```python
from build123d import *

# Parameters (mm, degrees)
SKETCH1_W           = 65.8
SKETCH1_H           = 130
BOSS_EXTRUDE1_DEPTH = 11.4
CUT_EXTRUDE1_DEPTH  = 94.191201301
FILLET1_R           = 11
SKETCH3_R           = 5.5
SKETCH3_R_2         = 2.75
CUT_EXTRUDE2_DEPTH  = 1
SKETCH4_W           = 16
SKETCH4_H           = 1.3
SKETCH4_W_2         = 9
BOSS_EXTRUDE2_DEPTH = 1
SKETCH5_W           = 7.2
SKETCH5_H           = 2
CUT_EXTRUDE3_DEPTH  = 1
FILLET2_R           = 0.5
FILLET3_R           = 1.5


with BuildPart() as part:
    # Sketch1 → Boss-Extrude1 (new body)
    with BuildSketch(Plane(origin=(0, 0, 0), x_dir=(1, 0, 0), z_dir=(0, 1, 0))):
        Rectangle(SKETCH1_W, SKETCH1_H)
    extrude(amount=BOSS_EXTRUDE1_DEPTH)

    # Sketch2 → Cut-Extrude1 (cut, through all)
    with BuildSketch(Plane(origin=(32.9, 0, 0), x_dir=(0, 0, -1), z_dir=(1, 0, 0))):
        with BuildLine():
            Line((-65, 2.7), (-65, 0))
            Line((-65, 0), (0, 0))
            ThreePointArc((0, 0), (-32.528026377, 0.675290918), (-65, 2.7))
        make_face()
    extrude(amount=-CUT_EXTRUDE1_DEPTH, mode=Mode.SUBTRACT)

    # Fillet1
    fillet1_edges = [part.edges().sort_by_distance(p)[0] for p in [
        (32.9, 7.05, 65),
        (-32.9, 7.05, 65),
        (-32.9, 5.7, -65),
        (32.9, 5.7, -65),
    ]]
    fillet(fillet1_edges, radius=FILLET1_R)

    # Sketch3 → Cut-Extrude2 (cut)
    with BuildSketch(Plane.XZ):
        with Locations(Location((0, -44.1, 0), (0, 0, 270))):
            Circle(SKETCH3_R)
        with Locations(Location((0, -30.7, 0), (0, 0, 270))):
            Circle(SKETCH3_R_2)
    extrude(amount=-CUT_EXTRUDE2_DEPTH, mode=Mode.SUBTRACT)

    # Sketch4 → Boss-Extrude2 (add)
    with BuildSketch(Plane(origin=(32.9, 0, 0), x_dir=(0, 0, -1), z_dir=(1, 0, 0))):
        with Locations((11, 7.75)):
            Rectangle(SKETCH4_W, SKETCH4_H)
        with Locations((35.5, 7.75)):
            Rectangle(SKETCH4_W_2, SKETCH4_H)
    extrude(amount=BOSS_EXTRUDE2_DEPTH)

    # Sketch5 → Cut-Extrude3 (cut)
    with BuildSketch(Plane.XY.offset(65)):
        with Locations((0, 7.05)):
            Rectangle(SKETCH5_W, SKETCH5_H)
    extrude(amount=-CUT_EXTRUDE3_DEPTH, mode=Mode.SUBTRACT)

    # Fillet2
    fillet2_edges = [part.edges().sort_by_distance(p)[0] for p in [
        (33.4, 7.1, -19),
        (33.4, 8.4, -19),
        (33.4, 8.4, -3),
        (33.4, 7.1, -3),
        (33.4, 7.1, -40),
        (33.4, 8.4, -40),
        (33.4, 8.4, -31),
        (33.4, 7.1, -31),
    ]]
    fillet(fillet2_edges, radius=FILLET2_R)

    # Fillet3
    fillet3_edges = [part.edges().sort_by_distance(p)[0] for p in [
        (32.9, 0, -27),
        (-32.9, 0.465759006, 27.016054675),
        (32.9, 0.465759006, 27.016054675),
        (-32.9, 0, -27),
        (-32.9, 11.4, 0),
        (0, 0, -65),
        (29.678174593, 0, -61.778174593),
        (-29.678174593, 0, -61.778174593),
        (0, 11.4, -65),
        (32.9, 11.4, 0),
        (0, 11.4, 65),
        (-29.678174593, 11.4, 61.778174593),
        (29.678174593, 11.4, 61.778174593),
        (29.678174593, 11.4, -61.778174593),
        (-29.678174593, 11.4, -61.778174593),
        (0, 2.7, 65),
        (-29.683166447, 2.438171783, 61.773179536),
        (29.683166447, 2.438171783, 61.773179536),
    ]]
    fillet(fillet3_edges, radius=FILLET3_R)


solid = part.part
```
Input: part model. Units: mm. Frame: model coordinates. A direction names the side the tool comes from. Give positions to 0.01 mm unless a question says otherwise; leave off trailing zeros. Order: outer loops, then holes, each group sorted by start corner. A loop starts at its lowest first (then second) coordinate and runs counter-clockwise, first axis right, second up. Notation, with made-up numbers: M 38,50.25 L 83,50.25 A28 ccw 83,89.25 Z; hole C 17.25,10 d8. An arc over 180 degrees is marked long. Return JSON: item names as keys, results as strings.
Item 1: Ray query, probe 1 along X at (y, z) = (3.75, -14); probe 2 along X at (y, z) = (0.65, -44.1); probe 3 along Y at (x, z) = (-8.5, 0.5). Return the intervals inside material, ascending.
Solutions:
{"probe 1": "-32.9 to 32.9", "probe 2": "-32.64 to -5.5, 5.5 to 32.64", "probe 3": "0 to 11.4"}
Item 2: Cut plane D-D (z = -13.5). Return loops of the section in (x, y), then the cut area to 3 significant figures.
Solutions:
{"outline": "M -32.9,1.5 A1.5 ccw -31.4,0 L 31.4,0 A1.5 ccw 32.9,1.5 L 32.9,7.1 L 33.9,7.1 L 33.9,8.4 L 32.9,8.4 L 32.9,9.9 A1.5 ccw 31.4,11.4 L -31.4,11.4 A1.5 ccw -32.9,9.9 Z", "area": "749 mm^2"}
Item 3: First-contact query: P1, Ø1, axis at x = -1, y = 7.5, coming from the +Z side; P2, Ø5.5, axis at x = -0.5, z = -44, coming from the -Y side; P3, Ø1.1, axis at x = 33.5, z = -14.5, coming from the -Y side. Flat tips, straight axial feed; report the tip coordinate or a pass-through.
Solutions:
{"P1": "z = 64", "P2": "y = 1", "P3": "y = 7.1"}
Item 4: Pull-direction query (Z, two-part tool) for faces 1 (the cylindrical face through (-29.763, 6.679, 61.692)), 2 (the flat face through (0, 1, -44)), 3 (the flat face through (0, 0, -25)); classes: +Z half, -Z half, draft (parallel to the pull), parting line (faces both ways), or undercut.
Solutions:
{"face 1": "+Z half", "face 2": "undercut", "face 3": "draft"}
Item 5: Cut plane A-A (x = 0). Return loops of the section in (y, z), then the cut area to 3 significant figures.
Solutions:
{"outline": "M 0,-63.5 A1.5 ccw 1.5,-65 L 9.9,-65 A1.5 ccw 11.4,-63.5 L 11.4,63.5 A1.5 ccw 9.9,65 L 8.05,65 L 8.05,64 L 6.05,64 L 6.05,65 L 4.08,65 A1.5 ccw 2.59,63.62 A783.76 ccw 0,0 L 0,-27.95 L 1,-27.95 L 1,-33.45 L 0,-33.45 L 0,-38.6 L 1,-38.6 L 1,-49.6 L 0,-49.6 Z", "area": "1,400 mm^2"}
Item 6: Cut plane C-C (x = 12). Return loops of the section in (y, z).
Solutions:
{"outline": "M 0,-63.5 A1.5 ccw 1.5,-65 L 9.9,-65 A1.5 ccw 11.4,-63.5 L 11.4,63.5 A1.5 ccw 9.9,65 L 4.08,65 A1.5 ccw 2.59,63.62 A783.76 ccw 0,0 Z"}
Item 7: Cut plane B-B (z = -44.1). Return loops of the section in (x, y), then the cut area to 3 significant figures.
Solutions:
{"outline": "M -32.9,1.5 A1.5 ccw -31.4,0 L -5.5,0 L -5.5,1 L 5.5,1 L 5.5,0 L 31.4,0 A1.5 ccw 32.9,1.5 L 32.9,9.9 A1.5 ccw 31.4,11.4 L -31.4,11.4 A1.5 ccw -32.9,9.9 Z", "area": "737 mm^2"}
Item 8: Access query for faces 4 (the cylindrical face through (-3.3, 0.5, -39.7)), 5 (the cylindrical face through (-29.763, 5.759, -61.692)). Directions: +Z, -Z, +X, -X, +Y, -Y. A direction counts if a zero-diameter tool reaches every point of the face in a straight line with its end or side. Return the directions, or none.
Solutions:
{"face 4": "-Y", "face 5": "-Z, -X, +Y, -Y"}
